```python
from build123d import *

# Parameters (mm, degrees)
SKETCH_1_W           = 120
SKETCH_1_H           = 120
SKETCH_1_W_2         = 28
SKETCH_1_H_2         = 50
BASE_PLATE_DEPTH     = 4
TABS2_START          = -5
TABS2_DEPTH          = 10
TABS2_2_OUTLINE_W    = 26
TABS2_2_OUTLINE_H    = 4
TABS2_2_DEPTH        = 1.41096
TABS2_START_2        = 5
TABS2_3_OUTLINE_W    = 26
TABS2_3_OUTLINE_H    = 4
TABS2_3_DEPTH        = 20
TABS2_START_3        = -13
TABS2_4_DEPTH        = 26
TABS2_5_DEPTH        = 26
HOLE1_DEPTH          = 116.108644332
HOLE1_DEPTH_BACK     = 116.108644332
SKETCH_10_R          = 4.05
SKETCH_12_W          = 8.2
SKETCH_12_H          = 8.2
HOLE2_DEPTH          = 4
FILLETS_R            = 10
SKETCH_11_R          = 4
OBLONG_HOLES_DEPTH   = 4
OBLONG_HOLES_2_DEPTH = 4
FILLETS2_DEPTH       = 4
FILLETS3_R           = 15


with BuildPart() as part:
    # Base Plate: sheet metal written as solids
    # Sketch 1 → Base Plate (new body)
    with BuildSketch(Plane.XY):
        with Locations((-35, 0)):
            Rectangle(SKETCH_1_W, SKETCH_1_H)
        Rectangle(SKETCH_1_W_2, SKETCH_1_H_2, mode=Mode.SUBTRACT)
    extrude(amount=-BASE_PLATE_DEPTH)

    # Tabs2: read off the stored shape, not the designer's step
    # Tabs2 outline → Tabs2 (cut)
    with BuildSketch(Plane.XY.offset(TABS2_START)):
        with BuildLine():
            ThreePointArc((-13, 34.1), (-13.5, 34.6), (-14, 34.1))
            Line((-14, 34.1), (-14, 25))
            Line((-14, 25), (-13, 25))
            Line((-13, 25), (-13, 34.1))
        make_face()
        with BuildLine():
            Line((-13, -25), (-14, -25))
            Line((-14, -25), (-14, -34.1))
            ThreePointArc((-14, -34.1), (-13.5, -34.6), (-13, -34.1))
            Line((-13, -34.1), (-13, -25))
        make_face()
        with BuildLine():
            Line((13, 34.1), (13, 25))
            Line((13, 25), (14, 25))
            Line((14, 25), (14, 34.1))
            ThreePointArc((14, 34.1), (13.5, 34.6), (13, 34.1))
        make_face()
        with BuildLine():
            Line((14, -25), (13, -25))
            Line((13, -25), (13, -34.1))
            ThreePointArc((13, -34.1), (13.5, -34.6), (14, -34.1))
            Line((14, -34.1), (14, -25))
        make_face()
    extrude(amount=TABS2_DEPTH, mode=Mode.SUBTRACT)

    # Tabs2 2 outline → Tabs2 2 (cut)
    with BuildSketch(Plane.XY.offset(TABS2_START)):
        with Locations((0, 27)):
            Rectangle(TABS2_2_OUTLINE_W, TABS2_2_OUTLINE_H)
        with Locations((0, -27)):
            Rectangle(TABS2_2_OUTLINE_W, TABS2_2_OUTLINE_H)
    extrude(amount=TABS2_2_DEPTH, mode=Mode.SUBTRACT)

    # Tabs2 4 outline → Tabs2 4 (cut)
    with BuildSketch(Plane.YZ.offset(TABS2_START_3)):
        with BuildLine():
            ThreePointArc((34, -4), (29.757359313, -2.937253933), (26.516685226, 0))
            Line((26.516685226, 0), (25, 0))
            Line((25, 0), (25, -3.58904))
            Line((25, -3.58904), (29, -3.58904))
            Line((29, -3.58904), (29, -4))
            Line((29, -4), (34, -4))
        make_face()
        with BuildLine():
            Line((-25, -3.58904), (-25, 0))
            Line((-25, 0), (-26.516685226, 0))
            ThreePointArc((-26.516685226, 0), (-29.757359313, -2.937253933), (-34, -4))
            Line((-34, -4), (-29, -4))
            Line((-29, -4), (-29, -3.58904))
            Line((-29, -3.58904), (-25, -3.58904))
        make_face()
    extrude(amount=TABS2_4_DEPTH, mode=Mode.SUBTRACT)



with BuildPart() as body_2:
    # Tabs2 3 outline → Tabs2 3 (new body)
    with BuildSketch(Plane.XY.offset(TABS2_START_2)):
        with Locations((0, 27)):
            Rectangle(TABS2_3_OUTLINE_W, TABS2_3_OUTLINE_H)
        with Locations((0, -27)):
            Rectangle(TABS2_3_OUTLINE_W, TABS2_3_OUTLINE_H)
    extrude(amount=TABS2_3_DEPTH)


with BuildPart() as part_1:
    add(part.part)

    add(body_2.part)  # Tabs2 5 merges body 2
    # Tabs2 5 outline → Tabs2 5 (add)
    with BuildSketch(Plane.YZ.offset(TABS2_START_3)):
        with BuildLine():
            Line((29, 5), (25, 5))
            ThreePointArc((25, 5), (25.38751392, 2.38751392), (26.516685226, 0))
            Line((26.516685226, 0), (34, 0))
            ThreePointArc((34, 0), (30.464466094, 1.464466094), (29, 5))
        make_face()
        with BuildLine():
            Line((-34, 0), (-26.516685226, 0))
            ThreePointArc((-26.516685226, 0), (-25.38751392, 2.38751392), (-25, 5))
            Line((-25, 5), (-29, 5))
            ThreePointArc((-29, 5), (-30.464466094, 1.464466094), (-34, 0))
        make_face()
    extrude(amount=TABS2_5_DEPTH)

    # Эскиз10 → Hole1 (cut, two sides: drawn at the far end of the back side and taken through both)
    with BuildSketch(Plane(origin=(0, 0, 0), x_dir=(1, 0, 0), z_dir=(0, 1, 0)).offset(-HOLE1_DEPTH_BACK)):
        with Locations(Location((0, -17, 0), (0, 0, 90))):
            Circle(SKETCH_10_R)
    extrude(amount=HOLE1_DEPTH + HOLE1_DEPTH_BACK, mode=Mode.SUBTRACT)

    # Эскиз12 → Hole2 (cut)
    with BuildSketch(Plane(origin=(0, 29, 0), x_dir=(1, 0, 0), z_dir=(0, 1, 0))):
        with Locations((0, -17)):
            Rectangle(SKETCH_12_W, SKETCH_12_H)
    extrude(amount=-HOLE2_DEPTH, mode=Mode.SUBTRACT)

    # Fillets
    fillets_edges = [part_1.edges().sort_by_distance(p)[0] for p in [
        (13, -27, 25),
        (-13, -27, 25),
        (-95, 60, -2),
        (25, 60, -2),
        (25, -60, -2),
        (-95, -60, -2),
        (-13, 27, 25),
        (13, 27, 25),
    ]]
    fillet(fillets_edges, radius=FILLETS_R)

    # Эскиз11 → Oblong Holes (cut)
    with BuildSketch(Plane.XY):
        with Locations((-86, 51)):
            Circle(SKETCH_11_R)
        with Locations((16, 51)):
            Circle(SKETCH_11_R)
        with Locations((-86, -51)):
            Circle(SKETCH_11_R)
        with Locations((16, -51)):
            Circle(SKETCH_11_R)
    extrude(amount=-OBLONG_HOLES_DEPTH, mode=Mode.SUBTRACT)

    # Эскиз13 → oblong Holes 2 (cut)
    with BuildSketch(Plane.XY):
        with BuildLine():
            Line((-83.171572875, 53.828427125), (-79.636038969, 50.292893219))
            ThreePointArc((-79.636038969, 50.292893219), (-79.636038969, 44.636038969), (-85.292893219, 44.636038969))
            Line((-85.292893219, 44.636038969), (-88.828427125, 48.171572875))
            ThreePointArc((-88.828427125, 48.171572875), (-88.828427125, 53.828427125), (-83.171572875, 53.828427125))
        make_face()
        with BuildLine():
            Line((18.828427125, 48.171572875), (15.292893219, 44.636038969))
            ThreePointArc((15.292893219, 44.636038969), (9.636038969, 44.636038969), (9.636038969, 50.292893219))
            Line((9.636038969, 50.292893219), (13.171572875, 53.828427125))
            ThreePointArc((13.171572875, 53.828427125), (18.828427125, 53.828427125), (18.828427125, 48.171572875))
        make_face()
        with BuildLine():
            Line((-88.828427125, -48.171572875), (-85.292893219, -44.636038969))
            ThreePointArc((-85.292893219, -44.636038969), (-79.636038969, -44.636038969), (-79.636038969, -50.292893219))
            Line((-79.636038969, -50.292893219), (-83.171572875, -53.828427125))
            ThreePointArc((-83.171572875, -53.828427125), (-88.828427125, -53.828427125), (-88.828427125, -48.171572875))
        make_face()
        with BuildLine():
            Line((13.171572875, -53.828427125), (9.636038969, -50.292893219))
            ThreePointArc((9.636038969, -50.292893219), (9.636038969, -44.636038969), (15.292893219, -44.636038969))
            Line((15.292893219, -44.636038969), (18.828427125, -48.171572875))
            ThreePointArc((18.828427125, -48.171572875), (18.828427125, -53.828427125), (13.171572875, -53.828427125))
        make_face()
    extrude(amount=-OBLONG_HOLES_2_DEPTH, mode=Mode.SUBTRACT)

    # Эскиз14 → Fillets2 (cut)
    with BuildSketch(Plane.XY):
        with BuildLine():
            Line((-95, 40), (-95, -40))
            ThreePointArc((-95, -40), (-75, 0), (-95, 40))
        make_face()
    extrude(amount=-FILLETS2_DEPTH, mode=Mode.SUBTRACT)

    # Fillets3
    fillets3_edges = [part_1.edges().sort_by_distance(p)[0] for p in [
        (-95, 40, -2),
        (-95, -40, -2),
    ]]
    fillet(fillets3_edges, radius=FILLETS3_R)


solid = part_1.part
```
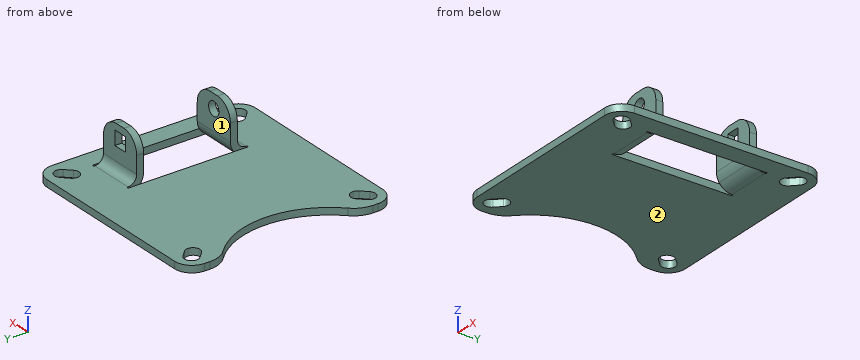
Here's how the part is built. I have some questions about the finished solid (model axes, mm). Face numbers are marked on the shaded views. A direction names the side the tool comes from. Coordinates: 2 decimals unless noted, no trailing zeros. Loops run counter-clockwise (first coordinate to the right, second up) from the corner with the lowest first, then second, coordinate; pieces in that order, holes last. Notation, with made-up numbers: (43, -29) - (63, -29) arc R26 ccw to (63, -11) - close; hole circle Ø3 at (12, 21). An arc over 180 degrees is marked (long way). Return JSON: item names as keys, results as strings. Group by question number.
Item 1: If we section it at D-D on x = -52: Write out the boundary of the cut face in (y, z).
Item 2: On a 3-axis mill with a long thin cutter (end or side, diameter ignored), from which of +Z, -Z, +X, -X, +Y, -Y can I reach the whole of each face in a straight line? I mean the marked faces 1 and 2. Say none if no direction works.
Item 3: If we section it at C-C on y = 2.5: Write out the boundary of the cut face in (x, z).
Item 4: Will these pins go through, and if not, where does the flat tip stop? P1, Ø6, axis at x = 4.5, z = 12.5, coming from the -Y side; P2, Ø3, axis at y = 27.5, z = 16, coming from the -X side; P3, Ø6.5, axis at x = 0, z = 17, coming from the -Y side; P4, Ø1, axis at x = -11.5, z = 6.5, coming from the +Y side.
Item 5: If we section it at A-A on z = 9.75: Write out the boundary of the cut face in (x, y), and give its area (3 significant figures).
Item 6: I need wall thicknesses on line 1 (Z direction, x = -62, y = 36); line 2 (X direction, y = -27.05, z = 17); line 3 (Y direction, x = 1, z = -1). Which ranges of each line are inside material? Lowest first, please. Write a range as from..to.
Item 7: If we section it at B-B on z = 17: Write out the boundary of the cut face in (x, y).
Calculated:
{
 "1": {"outline": "(-60, -4) - (60, -4) - (60, 0) - (-60, 0) - close"},
 "2": {"face 1": "+Z, -Z, +X, -X", "face 2": "-Z, +X, -X, +Y, -Y"},
 "3": {"outline": "(-75.06, -4) - (-14, -4) - (-14, 0) - (-75.06, 0) - close; (14, -4) - (25, -4) - (25, 0) - (14, 0) - close"},
 "4": {"P1": "stops at y = -29", "P2": "stops at x = -13", "P3": "passes through", "P4": "stops at y = 29"},
 "5": {"outline": "(-13, -29) - (13, -29) - (13, -25) - (-13, -25) - close; (-13, 25) - (13, 25) - (13, 29) - (-13, 29) - close", "area": "208 mm^2"},
 "6": {"line 1": "z = -4..0", "line 2": "x = -12.8..-4.05, 4.05..12.8", "line 3": "y = -60..-27.29, 27.29..60"},
 "7": {"outline": "(-12.8, -29) - (-4.05, -29) - (-4.05, -25) - (-12.8, -25) - close; (-12.8, 25) - (-4.1, 25) - (-4.1, 29) - (-12.8, 29) - close; (4.05, -29) - (12.8, -29) - (12.8, -25) - (4.05, -25) - close; (4.1, 25) - (12.8, 25) - (12.8, 29) - (4.1, 29) - close"}
}
